```python
from build123d import *

# Parameters (mm, degrees)
SKETCH_1_W           = 15
SKETCH_1_H           = 15
SKETCH_1_W_2         = 12
SKETCH_1_H_2         = 12
EXTRUDE_2_DEPTH      = 144
SKETCH_3_R           = 1.5
CUT_EXTRUDE_2_DEPTH  = 10
SKETCH_4_R           = 1.5
CUT_EXTRUDE_4_DEPTH  = 10
SKETCH_7_R           = 4
CUT_EXTRUDE_6_DEPTH  = 10
SKETCH_8_R           = 4
CUT_EXTRUDE_7_DEPTH  = 10
SKETCH_9_R           = 6
CUT_EXTRUDE_8_DEPTH  = 10
SKETCH_10_R          = 1.5
CUT_EXTRUDE_9_DEPTH  = 10
SKETCH_11_R          = 4
CUT_EXTRUDE_10_DEPTH = 10
SKETCH_12_R          = 6
CUT_EXTRUDE_11_DEPTH = 10
SKETCH_13_R          = 1.5
CUT_EXTRUDE_12_DEPTH = 10
SKETCH_14_R          = 1.5
CUT_EXTRUDE_13_DEPTH = 10
SKETCH_15_R          = 1.5
CUT_EXTRUDE_14_DEPTH = 10


with BuildPart() as part:
    # ｽｹｯﾁ1 → ﾎﾞｽ - 押し出し2 (new body)
    with BuildSketch(Plane.XY):
        with Locations((0.489915859, 0.232626086)):
            Rectangle(SKETCH_1_W, SKETCH_1_H)
        with Locations((0.489915859, 0.232626086)):
            Rectangle(SKETCH_1_W_2, SKETCH_1_H_2, mode=Mode.SUBTRACT)
    extrude(amount=EXTRUDE_2_DEPTH)

    # ｽｹｯﾁ3 → ｶｯﾄ - 押し出し2 (cut)
    with BuildSketch(Plane(origin=(0, 7.732626086, 0), x_dir=(1, 0, 0), z_dir=(0, 1, 0))):
        with Locations((0.489915859, -22.5)):
            Circle(SKETCH_3_R)
    extrude(amount=-CUT_EXTRUDE_2_DEPTH, mode=Mode.SUBTRACT)

    # ｽｹｯﾁ4 → ｶｯﾄ - 押し出し4 (cut)
    with BuildSketch(Plane(origin=(0, 7.732626086, 0), x_dir=(1, 0, 0), z_dir=(0, 1, 0))):
        with Locations((0.489915859, -121.5)):
            Circle(SKETCH_4_R)
    extrude(amount=-CUT_EXTRUDE_4_DEPTH, mode=Mode.SUBTRACT)

    # ｽｹｯﾁ7 → ｶｯﾄ - 押し出し6 (cut)
    with BuildSketch(Plane.XZ.offset(7.267373914)):
        with Locations((0.489915859, 22.5)):
            Circle(SKETCH_7_R)
    extrude(amount=-CUT_EXTRUDE_6_DEPTH, mode=Mode.SUBTRACT)

    # ｽｹｯﾁ8 → ｶｯﾄ - 押し出し7 (cut)
    with BuildSketch(Plane.XZ.offset(7.267373914)):
        with Locations((0.489915859, 121.5)):
            Circle(SKETCH_8_R)
    extrude(amount=-CUT_EXTRUDE_7_DEPTH, mode=Mode.SUBTRACT)

    # ｽｹｯﾁ9 → ｶｯﾄ - 押し出し8 (cut)
    with BuildSketch(Plane.ZY.offset(7.010084141)):
        with Locations((37.5, 0.232626086)):
            Circle(SKETCH_9_R)
    extrude(amount=-CUT_EXTRUDE_8_DEPTH, mode=Mode.SUBTRACT)

    # ｽｹｯﾁ10 → ｶｯﾄ - 押し出し9 (cut)
    with BuildSketch(Plane(origin=(7.989915859, 0, 0), x_dir=(0, 0, -1), z_dir=(1, 0, 0))):
        with Locations((-37.5, 0.232626086)):
            Circle(SKETCH_10_R)
    extrude(amount=-CUT_EXTRUDE_9_DEPTH, mode=Mode.SUBTRACT)

    # ｽｹｯﾁ11 → ｶｯﾄ - 押し出し10 (cut)
    with BuildSketch(Plane.XZ.offset(7.267373914)):
        with Locations((0.489915859, 72.5)):
            Circle(SKETCH_11_R)
    extrude(amount=-CUT_EXTRUDE_10_DEPTH, mode=Mode.SUBTRACT)

    # ｽｹｯﾁ12 → ｶｯﾄ - 押し出し11 (cut)
    with BuildSketch(Plane.ZY.offset(7.010084141)):
        with Locations((106.5, 0.232626086)):
            Circle(SKETCH_12_R)
    extrude(amount=-CUT_EXTRUDE_11_DEPTH, mode=Mode.SUBTRACT)

    # ｽｹｯﾁ13 → ｶｯﾄ - 押し出し12 (cut)
    with BuildSketch(Plane(origin=(7.989915859, 0, 0), x_dir=(0, 0, -1), z_dir=(1, 0, 0))):
        with Locations((-106.5, 0.232626086)):
            Circle(SKETCH_13_R)
    extrude(amount=-CUT_EXTRUDE_12_DEPTH, mode=Mode.SUBTRACT)

    # ｽｹｯﾁ14 → ｶｯﾄ - 押し出し13 (cut)
    with BuildSketch(Plane(origin=(7.989915859, 0, 0), x_dir=(0, 0, -1), z_dir=(1, 0, 0))):
        with Locations((-7.5, 0.232626086)):
            Circle(SKETCH_14_R)
    extrude(amount=-CUT_EXTRUDE_13_DEPTH, mode=Mode.SUBTRACT)

    # ｽｹｯﾁ15 → ｶｯﾄ - 押し出し14 (cut)
    with BuildSketch(Plane(origin=(7.989915859, 0, 0), x_dir=(0, 0, -1), z_dir=(1, 0, 0))):
        with Locations((-72.5, 0.232626086)):
            Circle(SKETCH_15_R)
    extrude(amount=-CUT_EXTRUDE_14_DEPTH, mode=Mode.SUBTRACT)


solid = part.part
```
Input: part model. Units: mm. Frame: model coordinates. A direction names the side the tool comes from. Round coordinates to 2 decimals unless told otherwise and drop trailing zeros. Loops run counter-clockwise (first coordinate to the right, second up) from the corner with the lowest first, then second, coordinate; pieces in that order, holes last. Notation, with made-up numbers: M 84.5,-22 L 131.5,-22 A8 ccw 131.5,-17 Z; hole C 5.5,19 d10. An arc over 180 degrees is marked long. Answer in a Markdown table with one row per item. Add a question column.
1. Set-up query: faces 1 (the face through (-0.031, -6.528, 26.466)), 2 (the face through (-6.27, -3.42, 32.74)), 3 (the face through (7.25, 0.68, 71.07)), 4 (the face through (-5.51, 0, 72)). Return all of +Z, -Z, +X, -X, +Y, -Y with unobstructed straight access to the full face (end or side cutting, diameter ignored); none if empty.
2. Section C-C (x = 0.75). Output: boundary loops of the cut face in (y, z).
3. Mould query, pull axis X, two halves, no side actions, for faces 5 (the face through (7.3, 0.3, 9)), 6 (the face through (7.99, -2, 71)), 7 (the face through (-5.51, 0, 129)). Classes: released by +X, released by -X, zero draft, split by the parting line, or undercut.
4. Contact query for flat-ended pins moving along their axis: pin 1 (4 mm diameter, centred on y = 0.23, z = 37.5, fed in from -X); pin 2 (1 mm diameter, centred on x = 3.5, y = 5, fed in from +Z); pin 3 (5 mm diameter, centred on x = 0.49, z = 22.5, fed in from -Y); pin 4 (6 mm diameter, centred on y = -4.5, z = 110, fed in from -X). Output: stop coordinate, or through.
5. Ray query, probe 1 along Y at (x, z) = (-2.25, 16); probe 2 along Y at (x, z) = (7.5, 7.5); probe 3 along X at (y, z) = (4.5, 59). Return the intervals inside material, ascending.
6. Section D-D (z = 7.5). Output: boundary loops of the cut face in (x, y).
7. Section B-B (y = -4). Output: boundary loops of the cut face in (x, z), and give its area (3 significant figures).
8. Section A-A (z = 72.5). Output: boundary loops of the cut face in (x, y).
Values follow:
| question | item | result |
|---|---|---|
| 1 | face 1 | -Y |
| 1 | face 2 | -X |
| 1 | face 3 | +X |
| 1 | face 4 | +Z, -Z |
| 2 | outline | M -7.27,0 L -5.77,0 L -5.77,18.51 L -7.27,18.51 Z; M -7.27,26.49 L -5.77,26.49 L -5.77,68.51 L -7.27,68.51 Z; M -7.27,76.49 L -5.77,76.49 L -5.77,117.51 L -7.27,117.51 Z; M -7.27,125.49 L -5.77,125.49 L -5.77,144 L -7.27,144 Z; M 6.23,0 L 7.73,0 L 7.73,21.02 L 6.23,21.02 Z; M 6.23,23.98 L 7.73,23.98 L 7.73,120.02 L 6.23,120.02 Z; M 6.23,122.98 L 7.73,122.98 L 7.73,144 L 6.23,144 Z |
| 3 | face 5 | zero draft |
| 3 | face 6 | released by +X |
| 3 | face 7 | undercut |
| 4 | pin 1 | x = 6.49 |
| 4 | pin 2 | through |
| 4 | pin 3 | y = 6.23 |
| 4 | pin 4 | x = -7.01 |
| 5 | probe 1 | -7.27 to -5.77, 6.23 to 7.73 |
| 5 | probe 2 | -7.27 to -1.27, 1.73 to 7.73 |
| 5 | probe 3 | -7.01 to -5.51, 6.49 to 7.99 |
| 6 | outline | M -7.01,-7.27 L 7.99,-7.27 L 7.99,-1.27 L 6.49,-1.27 L 6.49,-5.77 L -5.51,-5.77 L -5.51,6.23 L 6.49,6.23 L 6.49,1.73 L 7.99,1.73 L 7.99,7.73 L -7.01,7.73 Z |
| 7 | outline | M -7.01,0 L -5.51,0 L -5.51,33.25 L -7.01,33.25 Z; M -7.01,41.75 L -5.51,41.75 L -5.51,102.25 L -7.01,102.25 Z; M -7.01,110.75 L -5.51,110.75 L -5.51,144 L -7.01,144 Z; M 6.49,0 L 7.99,0 L 7.99,144 L 6.49,144 Z |
| 7 | area | 406 mm^2 |
| 8 | outline | M -7.01,-7.27 L -3.51,-7.27 L -3.51,-5.77 L -5.51,-5.77 L -5.51,6.23 L 6.49,6.23 L 6.49,1.73 L 7.99,1.73 L 7.99,7.73 L -7.01,7.73 Z; M 4.49,-7.27 L 7.99,-7.27 L 7.99,-1.27 L 6.49,-1.27 L 6.49,-5.77 L 4.49,-5.77 Z |
